Part model, mm, in its own coordinate system. A direction names the side the tool comes from. Give positions to 0.01 mm unless a question says otherwise; leave off trailing zeros. Write each loop counter-clockwise with the first axis right and the second up, starting at its lowest first coordinate (ties: lowest second). Pieces come first, ordered by that corner, then holes.
from build123d import *

# Parameters (mm, degrees)
CROQUIS1_W              = 850
CROQUIS1_H              = 850
SALIENTE_EXTRUIR1_DEPTH = 700
VACIADO1_T              = -12.7
CROQUIS2_W              = 850
CROQUIS2_H              = 850
SALIENTE_EXTRUIR2_DEPTH = 200
CROQUIS3_W              = 150
CROQUIS3_H              = 50
CORTAR_EXTRUIR1_DEPTH   = 90
BARRER4_PROFILE_R       = 6.35
CORTAR_EXTRUIR2_REACH   = 1385.319
CROQUIS28_W             = 154.421889756
CROQUIS28_H             = 225.805379595


with BuildPart() as part:
    # Croquis1 → Saliente-Extruir1 (new body)
    with BuildSketch(Plane(origin=(0, 0, 0), x_dir=(1, 0, 0), z_dir=(0, 1, 0))):
        with Locations((425, 425)):
            Rectangle(CROQUIS1_W, CROQUIS1_H)
    extrude(amount=SALIENTE_EXTRUIR1_DEPTH)

    # Vaciado1
    vaciado1_openings = [part.faces().sort_by_distance(p)[0] for p in [
        (425, 700, -425),
        (425, 0, -425),
    ]]
    offset(amount=VACIADO1_T, openings=vaciado1_openings, kind=Kind.INTERSECTION)

    # Croquis2 → Saliente-Extruir2 (add)
    with BuildSketch(Plane.XZ):
        with Locations((425, -425)):
            Rectangle(CROQUIS2_W, CROQUIS2_H)
    extrude(amount=SALIENTE_EXTRUIR2_DEPTH)

    # Croquis3 → Cortar-Extruir1 (cut)
    with BuildSketch(Plane.XZ.offset(200)):
        with Locations((154.404863241, -80.611350772)):
            Rectangle(CROQUIS3_W, CROQUIS3_H)
        with Locations((695.595136759, -80.611350772)):
            Rectangle(CROQUIS3_W, CROQUIS3_H)
        with Locations((154.404863241, -769.388649228)):
            Rectangle(CROQUIS3_W, CROQUIS3_H)
        with Locations((695.595136759, -769.388649228)):
            Rectangle(CROQUIS3_W, CROQUIS3_H)
    extrude(amount=-CORTAR_EXTRUIR1_DEPTH, mode=Mode.SUBTRACT)

    # Croquis8 → Cortar-Recubrir1 section 0
    with BuildSketch(Plane(origin=(0, 0, 0), x_dir=(1, 0, 0), z_dir=(0, 1, 0))):
        with BuildLine():
            Line((12.7, 12.7), (837.3, 12.7))
            Line((837.3, 12.7), (837.3, 837.3))
            Line((837.3, 837.3), (12.7, 837.3))
            Line((12.7, 837.3), (12.7, 12.7))
        make_face()
    # Croquis6 → Cortar-Recubrir1 section 1
    with BuildSketch(Plane(origin=(0, -160, 0), x_dir=(-1, 0, 0), z_dir=(0, -1, 0))):
        with BuildLine():
            Line((-602.765132653, 12.7), (-442.765132653, 12.7))
            Line((-442.765132653, 12.7), (-442.765132653, 172.7))
            Line((-442.765132653, 172.7), (-602.765132653, 172.7))
            Line((-602.765132653, 172.7), (-602.765132653, 12.7))
        make_face()
    loft(mode=Mode.SUBTRACT)

    # Barrer4: sweep along a path in Croquis11
    with BuildLine(Plane(origin=(0, 680, 0), x_dir=(1, 0, 0), z_dir=(0, 1, 0))) as barrer4_path:
        Line((0, 248.298675653), (-70, 248.298675653))
        ThreePointArc((-70, 248.298675653), (-91.213203436, 257.085472217), (-100, 278.298675653))
        Line((-100, 278.298675653), (-100, 571.701324347))
        ThreePointArc((-100, 571.701324347), (-91.213203436, 592.914527783), (-70, 601.701324347))
        Line((-70, 601.701324347), (0, 601.701324347))
    # Barrer4 profile (on start of the path) → Barrer4 (sweep)
    with BuildSketch(Plane(origin=(0, 680, -248.298675653), x_dir=(0, 0, -1), z_dir=(-1, 0, 0))):
        Circle(BARRER4_PROFILE_R)
    sweep(path=barrer4_path.line)

    # Croquis28 → Cortar-Extruir2 (cut, up to next)
    with BuildSketch(Plane(origin=(0, 0, -12.7), x_dir=(-1, 0, 0), z_dir=(0, 0, -1)), mode=Mode.PRIVATE) as cortar_extruir2_sk1:
        with Locations((-525.554187775, -47.097310202)):
            Rectangle(CROQUIS28_W, CROQUIS28_H)
    cortar_extruir2_tool1 = extrude(cortar_extruir2_sk1.sketch, amount=-CORTAR_EXTRUIR2_REACH, mode=Mode.PRIVATE) & part.part
    add(cortar_extruir2_tool1.solids().sort_by_distance((525.554188, -47.09731, -12.7))[0], mode=Mode.SUBTRACT)


solid = part.part
1) Flat gauge pins, fed straight in: P1, Ø1.5, axis at y = 566, z = -285.5, coming from the -X side; P2, Ø25, axis at x = 175, z = -772.5, coming from the -Y side. Where does each tip first touch, or does it go through?
Check result:
P1: stops at x = 0
P2: stops at y = -110
2) Saw through at A-A (y = 339). Write the cut outline in (x, z), and give its area (3 significant figures).
Check result:
outline: (0, -850) - (850, -850) - (850, 0) - (0, 0) - close; hole (12.7, -837.3) - (837.3, -837.3) - (837.3, -12.7) - (12.7, -12.7) - close
area: 42,500 mm2
3) Drill centre lines: L1, parallel to X at y = 641.5, z = -359; L2, parallel to Z at x = 426, y = 220; L3, parallel to Y at x = 676.5, z = -290.5. Where is each one in solid material? Low to high.
Check result:
L1: x = 0 to 12.7, 837.3 to 850
L2: z = -850 to -837.3, -12.7 to 0
L3: y = -200 to -109.7
4) Saw through at B-B (y = 13). Write the cut outline in (x, z), and give its area (3 significant figures).
Check result:
outline: (0, -850) - (850, -850) - (850, 0) - (602.77, 0) - (602.77, -12.7) - (837.3, -12.7) - (837.3, -837.3) - (12.7, -837.3) - (12.7, -12.7) - (448.34, -12.7) - (448.34, 0) - (0, 0) - close
area: 40,600 mm2
5) 3-axis set-ups, long thin cutter, end or side, ignore diameter. For faces 1 (the flat face through (79.405, -156, -770)), 2 (the flat face through (620.595, -174, -81)), 3 (the flat face through (419, 345, -837.3)): which of +Z, -Z, +X, -X, +Y, -Y reach the whole face in a straight line?
Check result:
face 1: -Y
face 2: +Y, -Y
face 3: +Y
6) Mould opens along Z. For faces 4 (the flat face through (419, 256, 0)), 5 (the flat face through (419, -200, -419)), 6 (the flat face through (153, -110, -769)) say: +Z half, -Z half, draft (parallel to the pull), parting line (faces both ways), or undercut.
Check result:
face 4: +Z half
face 5: draft
face 6: undercut
